Drawing for the job (mm, zero at the part's lowest x, y, z). A direction names the side the tool comes from. Give positions to 0.01 mm unless a question says otherwise; leave off trailing zeros. Order: outer loops, then holes, each group sorted by start corner. A loop starts at its lowest first (then second) coordinate and runs counter-clockwise, first axis right, second up. Notation, with made-up numbers: (59.5, -36.5) -> (88.5, -36.5) arc R22 ccw to (88.5, -10.5) -> close; hole circle Ø1 at (72, 43.25). An arc over 180 degrees is marked (long way). Use one line per item in the form item = value. Start each with the question number.
1) Cut at C-C, the plane x = 47.5. Give the cut face in (y, z), and give its area (3 significant figures).
2) Probe line 1 (Y direction, x = 47.5, z = 86.5); line 2 (Y direction, x = 12.5, z = 2.4); line 3 (Z direction, x = 41, y = 12). List the from-to ranges inside material, lowest first.
3) Cut at B-B, the plane z = 45. Give the cut face in (x, y).
4) Cut at D-D, the plane z = 32. Give the cut face in (x, y), and give its area (3 significant figures).
5) Drop flat-ended pins along their axis: P1, Ø5.5, axis at x = 34, z = 88, coming from the -Y side; P2, Ø4, axis at x = 47.5, y = 22.5, coming from the +Z side; P3, Ø1.5, axis at x = 32, z = 88.5, coming from the +Y side. Give the stop position or say it passes through.
6) Tool access for the marked faces 4 and 5: list every direction of +Z, -Z, +X, -X, +Y, -Y with a clear straight run to the whole face (end or side of a thin tool).
7) Mould opens along Z. For the marked faces 1, 2 and 3 say: pulls with the +Z half, pulls with the -Z half, needs draft (parallel to the pull), parting line crosses it, or undercut.
8) Cut at A-A, the plane y = 40. Give the cut face in (x, z).
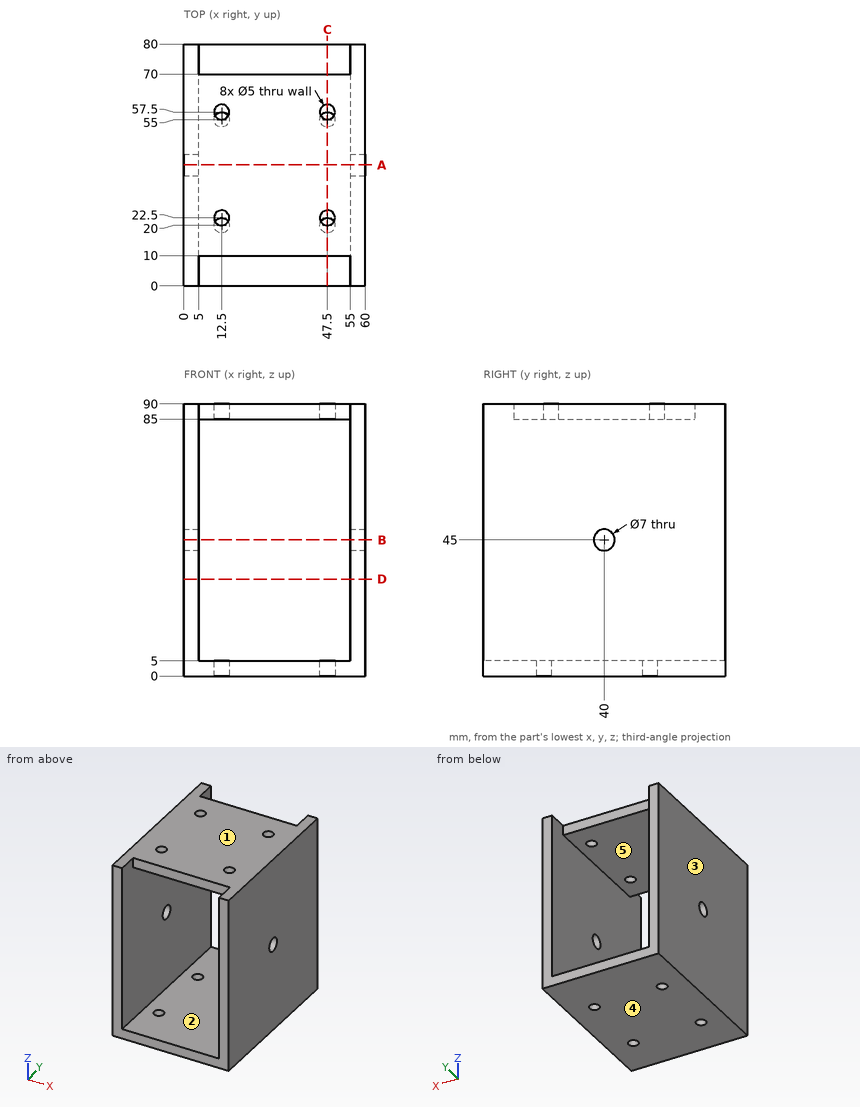
Result:
q1.outline = (0, 0) -> (17.5, 0) -> (17.5, 5) -> (0, 5) -> close; (10, 85) -> (20, 85) -> (20, 90) -> (10, 90) -> close; (22.5, 0) -> (52.5, 0) -> (52.5, 5) -> (22.5, 5) -> close; (25, 85) -> (55, 85) -> (55, 90) -> (25, 90) -> close; (57.5, 0) -> (80, 0) -> (80, 5) -> (57.5, 5) -> close; (60, 85) -> (70, 85) -> (70, 90) -> (60, 90) -> close
q1.area = 600 mm²
q2.line_1 = 10 to 20, 25 to 55, 60 to 70
q2.line_2 = 0 to 17.5, 22.5 to 52.5, 57.5 to 80
q2.line_3 = 0 to 5, 85 to 90
q3.outline = (0, 0) -> (5, 0) -> (5, 36.5) -> (0, 36.5) -> close; (0, 43.5) -> (5, 43.5) -> (5, 80) -> (0, 80) -> close; (55, 0) -> (60, 0) -> (60, 36.5) -> (55, 36.5) -> close; (55, 43.5) -> (60, 43.5) -> (60, 80) -> (55, 80) -> close
q4.outline = (0, 0) -> (5, 0) -> (5, 80) -> (0, 80) -> close; (55, 0) -> (60, 0) -> (60, 80) -> (55, 80) -> close
q4.area = 800 mm²
q5.P1 = 10
q5.P2 = 5
q5.P3 = 70
q6.face_4 = -Z, +X, -X, +Y, -Y
q6.face_5 = +Y, -Y
q7.face_1 = pulls with the +Z half
q7.face_2 = undercut
q7.face_3 = needs draft
q8.outline = (0, 0) -> (60, 0) -> (60, 41.5) -> (55, 41.5) -> (55, 5) -> (5, 5) -> (5, 41.5) -> (0, 41.5) -> close; (0, 48.5) -> (5, 48.5) -> (5, 85) -> (55, 85) -> (55, 48.5) -> (60, 48.5) -> (60, 90) -> (0, 90) -> close
